Input: dimensioned drawing with shaded views. Units: mm. Origin: part minimum x, y, z. Round coordinates to 2 decimals unless told otherwise and drop trailing zeros. Order: outer loops, then holes, each group sorted by start corner. A loop starts at its lowest first (then second) coordinate and runs counter-clockwise, first axis right, second up. Notation, with made-up numbers: M -8.75,88.25 L 16.25,88.25 A11 ccw 16.25,105.25 Z; hole C 32,75 d2. An arc over 180 degrees is marked long. One line per question, with ' | ' between items.
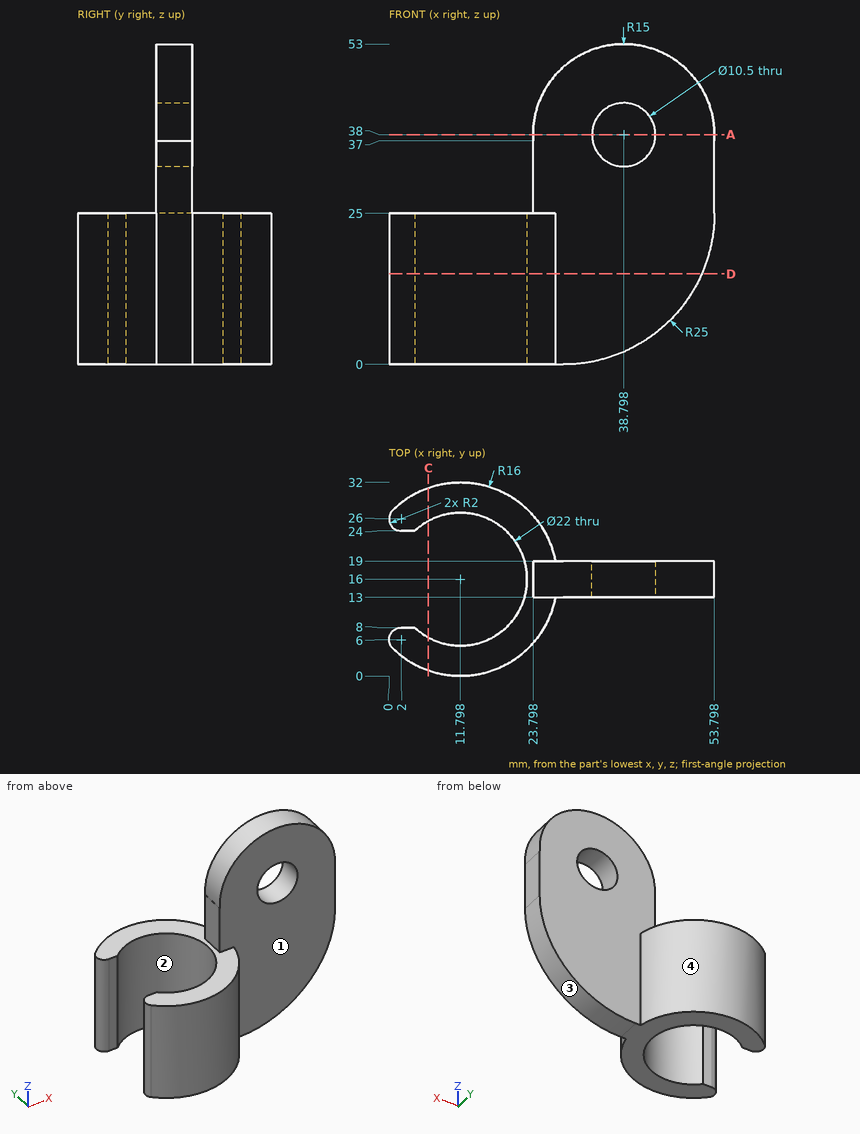
Item 1: Mould query, pull axis X, two halves, no side actions, for the marked faces 1, 2, 3 and 4. Classes: +X half, -X half, draft (parallel to the pull), parting line (faces both ways), or undercut.
Report:
face 1: draft | face 2: undercut | face 3: +X half | face 4: parting line
Item 2: Section query A-A, the plane z = 38. Return loops of the section in (x, y), plus the area to 3 significant figures.
Report:
outline: M 23.8,13 L 33.55,13 L 33.55,19 L 23.8,19 Z; M 44.05,13 L 53.8,13 L 53.8,19 L 44.05,19 Z | area: 117 mm²
Item 3: Section query C-C, the plane x = 6.5. Return loops of the section in (y, z).
Report:
outline: M 0.9,0 L 6.36,0 L 6.36,25 L 0.9,25 Z; M 25.64,0 L 31.1,0 L 31.1,25 L 25.64,25 Z
Item 4: Line query: line 1 along Z through (x, y) = (5, 7); line 2 along Y through (x, z) = (28, 33.5); line 3 along X through (y, z) = (16.5, 20). Output: solid intervals per line, ascending. Write a range as from..to.
Report:
line 1: 0..25 | line 2: 13..19 | line 3: 22.79..53.29
Item 5: Section query D-D, the plane z = 15. Return loops of the section in (x, y), plus the area to 3 significant figures.
Report:
outline: M 0.6,4.57 A16 ccw 27.51,13 L 51.71,13 L 51.71,19 L 27.51,19 A16 ccw 0.6,27.43 A2 ccw 2,24 L 4.25,24 A11 cw long 4.25,8 L 2,8 A2 ccw Z | area: 474 mm²
Item 6: First-contact query: pin 1 (6 mm diameter, centred on x = 46, y = 13, fed in from +Z); pin 2 (0.7 mm diameter, centred on x = 3.5, z = 7.5, fed in from +Y); pin 3 (3 mm diameter, centred on y = 15, z = 25, fed in from -X); pin 4 (12 mm diameter, centred on x = 14, z = 7.5, fed in from -Y). Flat tips, straight axial feed; report the tip coordinate or a pass-through.
Report:
pin 1: z = 52.4 | pin 2: y = 29.89 | pin 3: x = 22.51 | pin 4: y = 0
